Geometry: see drawing. Coordinates: mm, zero at the bounding-box minimum. Give positions to 0.01 mm unless a question says otherwise; leave off trailing zeros. Order: outer loops, then holes, each group sorted by start corner. A loop starts at its lowest first (then second) coordinate and runs counter-clockwise, first axis right, second up. Notation, with made-up numbers: (42.25, -26.5) - (97.25, -26.5) arc R14 ccw to (97.25, -4.5) - close; hole circle Ø8 at (7.5, -5). An arc over 180 degrees is marked (long way). Put each result on its own line as item: value. Start each with the question number.
1. Section D-D on x = 10.5. Return the cut outline in (y, z), plus the area to 3 significant figures.
2. Ray query, line 1 along Z through (x, y) = (27.5, 2.5); line 2 along Z through (x, y) = (17.5, 0.3); line 3 along X through (y, z) = (0.5, 23.5). Return the intervals inside material, ascending. Write a range as from..to.
3. Section B-B on y = 2.55. Return the cut outline in (x, z), plus the area to 3 significant figures.
4. Section A-A on x = 28.25. Return the cut outline in (y, z), plus the area to 3 significant figures.
5. Section C-C on z = 24.5. Return the cut outline in (x, y), plus the area to 3 significant figures.
6. First-contact query: P1, Ø1.5, axis at y = 0.5, z = 122.5, coming from the +X side. Flat tip, straight axial feed; report the tip coordinate or a pass-through.
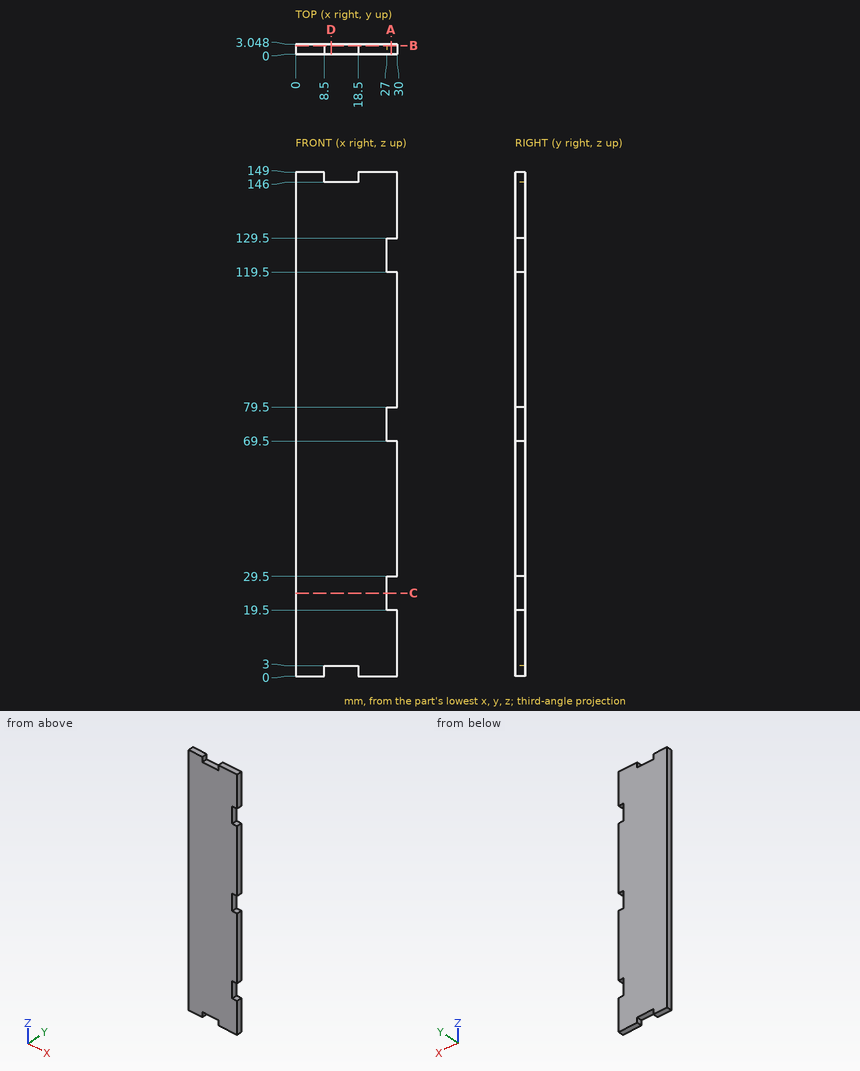
Resolved:
1. outline: (0, 3) - (3.05, 3) - (3.05, 146) - (0, 146) - close
1. area: 436 mm^2
2. line 1: 0..19.5, 29.5..69.5, 79.5..119.5, 129.5..149
2. line 2: 3..146
2. line 3: 0..27
3. outline: (0, 0) - (8.5, 0) - (8.5, 3) - (18.5, 3) - (18.5, 0) - (30, 0) - (30, 19.5) - (27, 19.5) - (27, 29.5) - (30, 29.5) - (30, 69.5) - (27, 69.5) - (27, 79.5) - (30, 79.5) - (30, 119.5) - (27, 119.5) - (27, 129.5) - (30, 129.5) - (30, 149) - (18.5, 149) - (18.5, 146) - (8.5, 146) - (8.5, 149) - (0, 149) - close
3. area: 4,320 mm^2
4. outline: (0, 0) - (3.05, 0) - (3.05, 19.5) - (0, 19.5) - close; (0, 29.5) - (3.05, 29.5) - (3.05, 69.5) - (0, 69.5) - close; (0, 79.5) - (3.05, 79.5) - (3.05, 119.5) - (0, 119.5) - close; (0, 129.5) - (3.05, 129.5) - (3.05, 149) - (0, 149) - close
4. area: 363 mm^2
5. outline: (0, 0) - (27, 0) - (27, 3.05) - (0, 3.05) - close
5. area: 82.3 mm^2
6. P1: x = 27
